The model under review builds one solid part; all positions refer to its coordinate system, in mm. A direction names the side the tool comes from. Coordinates: 2 decimals unless noted, no trailing zeros. Order: outer loops, then holes, each group sorted by start corner. A loop starts at its lowest first (then second) coordinate and runs counter-clockwise, first axis right, second up. Notation, with made-up numbers: (50, 3) -> (109, 3) arc R30 cw to (109, 39) -> close; hole circle Ø10 at (33, 24.5). An arc over 180 degrees is marked (long way). Put each result on its own line as item: value.
from build123d import *

# Parameters (mm, degrees)
SCHIZZO1_W                    = 74
SCHIZZO1_H                    = 60
ESTRUSIONE_ESTRUSIONE1_DEPTH  = 2
SCHIZZO2_W                    = 74
SCHIZZO2_H                    = 60
SCHIZZO2_W_2                  = 70
SCHIZZO2_H_2                  = 56
ESTRUSIONE_ESTRUSIONE2_DEPTH  = 18
SCHIZZO3_R                    = 1.7
TAGLIO_ESTRUSIONE1_DEPTH      = 8
SCHIZZO4_W                    = 68
SCHIZZO4_H                    = 8
TAGLIO_ESTRUSIONE2_DEPTH      = 56
TAGLIO_ESTRUSIONE2_DEPTH_BACK = 17
ESTRUSIONE_ESTRUSIONE3_DEPTH  = 27.5
SCHIZZO6_W                    = 2.5
SCHIZZO6_H                    = 25
ESTRUSIONE_ESTRUSIONE4_DEPTH  = 5
SCHIZZO7_W                    = 25
SCHIZZO7_H                    = 13
TAGLIO_ESTRUSIONE3_DEPTH      = 5
SCHIZZO8_W                    = 2
SCHIZZO8_H                    = 8
ESTRUSIONE_ESTRUSIONE5_DEPTH  = 9.5
SCHIZZO9_R                    = 1.25
ESTRUSIONE_ESTRUSIONE6_DEPTH  = 2.5


with BuildPart() as part:
    # Schizzo1 → Estrusione-Estrusione1 (new body)
    with BuildSketch(Plane(origin=(0, 0, 0), x_dir=(1, 0, 0), z_dir=(0, 1, 0))):
        Rectangle(SCHIZZO1_W, SCHIZZO1_H)
    extrude(amount=ESTRUSIONE_ESTRUSIONE1_DEPTH)

    # Schizzo2 → Estrusione-Estrusione2 (add)
    with BuildSketch(Plane(origin=(0, 2, 0), x_dir=(1, 0, 0), z_dir=(0, 1, 0))):
        Rectangle(SCHIZZO2_W, SCHIZZO2_H)
        Rectangle(SCHIZZO2_W_2, SCHIZZO2_H_2, mode=Mode.SUBTRACT)
    extrude(amount=ESTRUSIONE_ESTRUSIONE2_DEPTH)

    # Schizzo3 → Taglio-Estrusione1 (cut)
    with BuildSketch(Plane.XZ):
        with Locations((-30, 25)):
            Circle(SCHIZZO3_R)
        with Locations((30, 25)):
            Circle(SCHIZZO3_R)
        with Locations((30, -25)):
            Circle(SCHIZZO3_R)
        with Locations((-30, -25)):
            Circle(SCHIZZO3_R)
    extrude(amount=-TAGLIO_ESTRUSIONE1_DEPTH, mode=Mode.SUBTRACT)

    # Schizzo4 → Taglio-Estrusione2 (cut, two sides)
    with BuildSketch(Plane.XY.offset(-28)) as taglio_estrusione2_sk:
        with Locations((3, 16)):
            Rectangle(SCHIZZO4_W, SCHIZZO4_H)
    extrude(amount=TAGLIO_ESTRUSIONE2_DEPTH, mode=Mode.SUBTRACT)
    extrude(taglio_estrusione2_sk.sketch, amount=-TAGLIO_ESTRUSIONE2_DEPTH_BACK, mode=Mode.SUBTRACT)

    # Schizzo5 → Estrusione-Estrusione3 (add)
    with BuildSketch(Plane(origin=(0, 2, 0), x_dir=(1, 0, 0), z_dir=(0, 1, 0))):
        Polygon((-35, 21), (-29.5, 21), (-29.5, 15.569709151), (-29.5, 13), (-32, 13), (-32, 18.5), (-35, 18.5), align=None)
        Polygon((-29.5, -12), (-29.5, -6.768227203), (-29.5, -20), (-35, -20), (-35, -17.5), (-32, -17.5), (-32, -12), align=None)
    extrude(amount=ESTRUSIONE_ESTRUSIONE3_DEPTH)

    # Schizzo6 → Estrusione-Estrusione4 (add)
    with BuildSketch(Plane(origin=(0, 2, 0), x_dir=(1, 0, 0), z_dir=(0, 1, 0))):
        with Locations((-30.75, 0.5)):
            Rectangle(SCHIZZO6_W, SCHIZZO6_H)
    extrude(amount=ESTRUSIONE_ESTRUSIONE4_DEPTH)

    # Schizzo7 → Taglio-Estrusione3 (cut)
    with BuildSketch(Plane(origin=(-35, 0, 0), x_dir=(0, 0, -1), z_dir=(1, 0, 0))):
        with Locations((0.5, 13.5)):
            Rectangle(SCHIZZO7_W, SCHIZZO7_H)
    extrude(amount=-TAGLIO_ESTRUSIONE3_DEPTH, mode=Mode.SUBTRACT)

    # Schizzo8 → Estrusione-Estrusione5 (add)
    with BuildSketch(Plane(origin=(0, 20, 0), x_dir=(1, 0, 0), z_dir=(0, 1, 0))):
        with Locations((-36, 17)):
            Rectangle(SCHIZZO8_W, SCHIZZO8_H)
        with Locations((-36, -16)):
            Rectangle(SCHIZZO8_W, SCHIZZO8_H)
    extrude(amount=ESTRUSIONE_ESTRUSIONE5_DEPTH)

    # Schizzo9 → Estrusione-Estrusione6 (add)
    with BuildSketch(Plane.XZ):
        with BuildLine():
            Line((-37, -24.136555447), (-37, -19.136555447))
            Line((-37, -19.136555447), (-41.5, -19.136555447))
            ThreePointArc((-41.5, -19.136555447), (-44, -21.636555447), (-41.5, -24.136555447))
            Line((-41.5, -24.136555447), (-37, -24.136555447))
        make_face()
        with Locations((-41.5, -21.636555447)):
            Circle(SCHIZZO9_R, mode=Mode.SUBTRACT)
        with BuildLine():
            Line((-37, -2.5), (-37, 2.5))
            Line((-37, 2.5), (-41.5, 2.5))
            ThreePointArc((-41.5, 2.5), (-44, 0), (-41.5, -2.5))
            Line((-41.5, -2.5), (-37, -2.5))
        make_face()
        with Locations((-41.5, 0)):
            Circle(SCHIZZO9_R, mode=Mode.SUBTRACT)
        with BuildLine():
            Line((-37, 19.136555447), (-37, 24.136555447))
            Line((-37, 24.136555447), (-41.5, 24.136555447))
            ThreePointArc((-41.5, 24.136555447), (-44, 21.636555447), (-41.5, 19.136555447))
            Line((-41.5, 19.136555447), (-37, 19.136555447))
        make_face()
        with Locations((-41.5, 21.636555447)):
            Circle(SCHIZZO9_R, mode=Mode.SUBTRACT)
        with BuildLine():
            Line((37, 24.136555447), (37, 19.136555447))
            Line((37, 19.136555447), (41.5, 19.136555447))
            ThreePointArc((41.5, 19.136555447), (44, 21.636555447), (41.5, 24.136555447))
            Line((41.5, 24.136555447), (37, 24.136555447))
        make_face()
        with Locations((41.5, 21.636555447)):
            Circle(SCHIZZO9_R, mode=Mode.SUBTRACT)
        with BuildLine():
            Line((37, 2.5), (37, -2.5))
            Line((37, -2.5), (41.5, -2.5))
            ThreePointArc((41.5, -2.5), (44, 0), (41.5, 2.5))
            Line((41.5, 2.5), (37, 2.5))
        make_face()
        with Locations((41.5, 0)):
            Circle(SCHIZZO9_R, mode=Mode.SUBTRACT)
        with BuildLine():
            Line((37, -19.136555447), (37, -24.136555447))
            Line((37, -24.136555447), (41.5, -24.136555447))
            ThreePointArc((41.5, -24.136555447), (44, -21.636555447), (41.5, -19.136555447))
            Line((41.5, -19.136555447), (37, -19.136555447))
        make_face()
        with Locations((41.5, -21.636555447)):
            Circle(SCHIZZO9_R, mode=Mode.SUBTRACT)
    extrude(amount=-ESTRUSIONE_ESTRUSIONE6_DEPTH)


solid = part.part
Item 1: For faces 4 (the flat face through (39, 1, 2.5)), 5 (the flat face through (-39, 1, -19.137)), 6 (the flat face through (-37, 5, 0)), 7 (the flat face through (-35, 6, 0)), 8 (the flat face through (18, 12, -29)), list the 3-axis set-ups (+Z, -Z, +X, -X, +Y, -Y) from which the entire face can be reached by the end or side of a thin tool; tool diameter is ignored.
Answers below:
face 4: +X, +Y, -Y
face 5: -X, +Y, -Y
face 6: -X, +Y
face 7: +Y
face 8: -Z, +X, +Y
Item 2: For line 1 (X direction, y = 3.25, z = -15); line 2 (Z direction, x = -34.5, y = 28.25); line 3 (Z direction, x = -41.5, y = 1.05), list the stretches that pass through material, from the lowest coordinate up. Write a range as from..to.
Answers below:
line 1: -37..-35, -32..-29.5, 35..37
line 2: -21..-18.5, 17.5..20
line 3: -24.14..-22.89, -20.39..-19.14, -2.5..-1.25, 1.25..2.5, 19.14..20.39, 22.89..24.14
Item 3: For pin 1 Ø6 at (x, z) = (30.5, 7) entering from +Y; pin 2 Ø2 at (x, y) = (-39, 1.5) entering from -Z; pin 3 Ø6 at (y, z) = (19, 13.5) entering from -X, all flat-tipped, find the tip position at first contact; note any pin that passes through.
Answers below:
pin 1: y = 2
pin 2: z = -24.14
pin 3: x = -37
Item 4: Consider section D-D on z = -11.5. Write out the cut boundary in (x, y), and give its area (4 significant figures).
Answers below:
outline: (-37, 0) -> (37, 0) -> (37, 12) -> (35, 12) -> (35, 2) -> (-29.5, 2) -> (-29.5, 7) -> (-32, 7) -> (-32, 2) -> (-35, 2) -> (-35, 7) -> (-37, 7) -> close
area: 190.5 mm^2
Item 5: Mouldability with a two-part tool opening along Z and no side actions: class faces 1 (the flat face through (40, 2.5, 0)), 2 (the flat face through (-39, 1, -24.137)), 3 (the flat face through (-35, 11, 24)) as +Z half, -Z half, draft (parallel to the pull), parting line (faces both ways), or undercut.
Answers below:
face 1: draft
face 2: -Z half
face 3: undercut
Item 6: Consider section A-A on x = 30. Write out the cut boundary in (y, z).
Answers below:
outline: (0, -30) -> (12, -30) -> (12, -28) -> (2, -28) -> (2, -26.7) -> (0, -26.7) -> close; (0, -23.3) -> (2, -23.3) -> (2, 23.3) -> (0, 23.3) -> close; (0, 26.7) -> (2, 26.7) -> (2, 28) -> (20, 28) -> (20, 30) -> (0, 30) -> close
Item 7: Consider section C-C on y = 5.25. Write out the cut boundary in (x, z), and give its area (4 significant figures).
Answers below:
outline: (-37, -30) -> (37, -30) -> (37, 30) -> (-37, 30) -> close; hole (-35, -28) -> (35, -28) -> (35, 28) -> (-35, 28) -> (-35, 20) -> (-29.5, 20) -> (-29.5, -21) -> (-35, -21) -> close; hole (-35, -18.5) -> (-32, -18.5) -> (-32, 17.5) -> (-35, 17.5) -> close
area: 637.5 mm^2
Item 8: Consider section B-B on y = 27.25. Write out the cut boundary in (x, z), and give its area (3 significant figures).
Answers below:
outline: (-37, -21) -> (-29.5, -21) -> (-29.5, -13) -> (-32, -13) -> (-32, -18.5) -> (-35, -18.5) -> (-35, -13) -> (-37, -13) -> close; (-37, 12) -> (-35, 12) -> (-35, 17.5) -> (-32, 17.5) -> (-32, 12) -> (-29.5, 12) -> (-29.5, 20) -> (-37, 20) -> close
area: 87.0 mm^2
